Build history of the part. All positions in model axes, mm. Give positions to 0.01 mm unless a question says otherwise; leave off trailing zeros. Order: outer loops, then holes, each group sorted by start corner. A loop starts at its lowest first (then second) coordinate and runs counter-clockwise, first axis right, second up. Notation, with made-up numbers: (-13.75, 69) - (41.25, 69) arc R20 ccw to (41.25, 84) - close; hole circle Ø11 at (42, 33.5). An arc over 180 degrees is marked (long way). Write each question's results on one line, items separated by ' | '. Start each with the question number.
1) Cut at B-B on y = 16.5. List the corners of the cut face in (x, z).
2) Cut at C-C on y = 6. List the corners of the cut face in (x, z), plus the area to 3 significant figures.
3) Drop a flat-ended pin along its axis: pin 1 Ø3.5 at (x, y) = (-8, 11) entering from +Z. Give the stop position or say it passes through.
4) Cut at A-A on x = -6. List the corners of the cut face in (y, z).
5) Cut at D-D on z = 1.05. List the corners of the cut face in (x, y), plus the area to 3 significant figures.
6) Drill centre lines: line 1 along Y through (x, z) = (-6, 0.25); line 2 along Z through (x, y) = (-10.25, 4); line 3 along Y through (x, z) = (-8.75, 0.15). Where is each one in solid material? Low to high. Write a range as from..to.
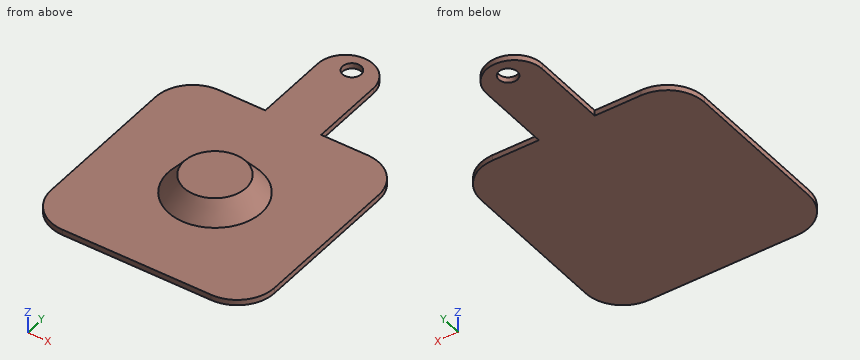
from build123d import *

# Parameters (mm, degrees)
EXTRUDE_1_DEPTH     = 0.3
FILLET_1_R          = 2
SKETCH_2_R          = 2.5
EXTRUDE_2_DEPTH     = 1
EXTRUDE_2_TAPER     = 40
SKETCH_3_R          = 0.5
CUT_EXTRUDE_1_DEPTH = 1


with BuildPart() as part:
    # 草图1 → 凸台-拉伸1 (new body)
    with BuildSketch(Plane.XY):
        with BuildLine():
            Line((-7.5, 12), (-12, 12))
            Line((-12, 12), (-12, 0))
            Line((-12, 0), (0, 0))
            Line((0, 0), (0, 12))
            Line((0, 12), (-4.5, 12))
            Line((-4.5, 12), (-4.5, 16))
            ThreePointArc((-4.5, 16), (-6, 17.5), (-7.5, 16))
            Line((-7.5, 16), (-7.5, 12))
        make_face()
    extrude(amount=EXTRUDE_1_DEPTH)

    # 圆角1
    fillet_1_edges = [part.edges().sort_by_distance(p)[0] for p in [
        (0, 0, 0.15),
        (-12, 0, 0.15),
        (-12, 12, 0.15),
        (0, 12, 0.15),
    ]]
    fillet(fillet_1_edges, radius=FILLET_1_R)

    # 草图2 → 凸台-拉伸2 (add)
    with BuildSketch(Plane.XY.offset(0.3)):
        with Locations((-6, 6)):
            Circle(SKETCH_2_R)
    extrude(amount=EXTRUDE_2_DEPTH, taper=EXTRUDE_2_TAPER)

    # 草图3 → 切除-拉伸1 (cut)
    with BuildSketch(Plane.XY.offset(0.3)):
        with Locations((-6, 16.5)):
            Circle(SKETCH_3_R)
    extrude(amount=-CUT_EXTRUDE_1_DEPTH, mode=Mode.SUBTRACT)


solid = part.part
Results:
1) outline: (-7.41, 0) - (-6.5, 0) - (-6.5, 0.3) - (-7.41, 0.3) - close; (-5.5, 0) - (-4.59, 0) - (-4.59, 0.3) - (-5.5, 0.3) - close
2) outline: (-12, 0) - (0, 0) - (0, 0.3) - (-3.5, 0.3) - (-4.34, 1.3) - (-7.66, 1.3) - (-8.5, 0.3) - (-12, 0.3) - close | area: 7.76 mm^2
3) pin 1: z = 0.3
4) outline: (0, 0) - (16, 0) - (16, 0.3) - (8.5, 0.3) - (7.66, 1.3) - (4.34, 1.3) - (3.5, 0.3) - (0, 0.3) - close; (17, 0) - (17.5, 0) - (17.5, 0.3) - (17, 0.3) - close
5) outline: circle Ø3.74 at (-6, 6) | area: 11.0 mm^2
6) line 1: 0..16, 17..17.5 | line 2: 0..0.3 | line 3: 0..12
